Verification items for this drawing (mm, ordinates from the low corner). Round coordinates to 2 decimals unless told otherwise and drop trailing zeros. Order: outer loops, then holes, each group sorted by start corner. A loop starts at its lowest first (then second) coordinate and runs counter-clockwise, first axis right, second up. Notation, with made-up numbers: (-16.5, 12) -> (28.5, 12) arc R22 cw to (28.5, 22) -> close; hole circle Ø4 at (-6, 75). An arc over 180 degrees is marked (long way). Return JSON: item names as keys, results as strings. Group by question number.
Item 1: Sectioned sample at A-A on x = 4. Record the cut outline in (y, z), plus the area to 3 significant figures.
Item 2: Sectioned sample at B-B on z = 0.65. Record the cut outline in (x, y).
Item 3: Sectioned sample at C-C on y = 69.5. Record the cut outline in (x, z).
Item 4: Scan lines: probe 1 along Y at (x, z) = (4.25, 0.4); probe 2 along X at (y, z) = (4, 0.7); probe 3 along X at (y, z) = (73, 0.35). Record each from-to range of solid material in increasing order. Write a range as from..to.
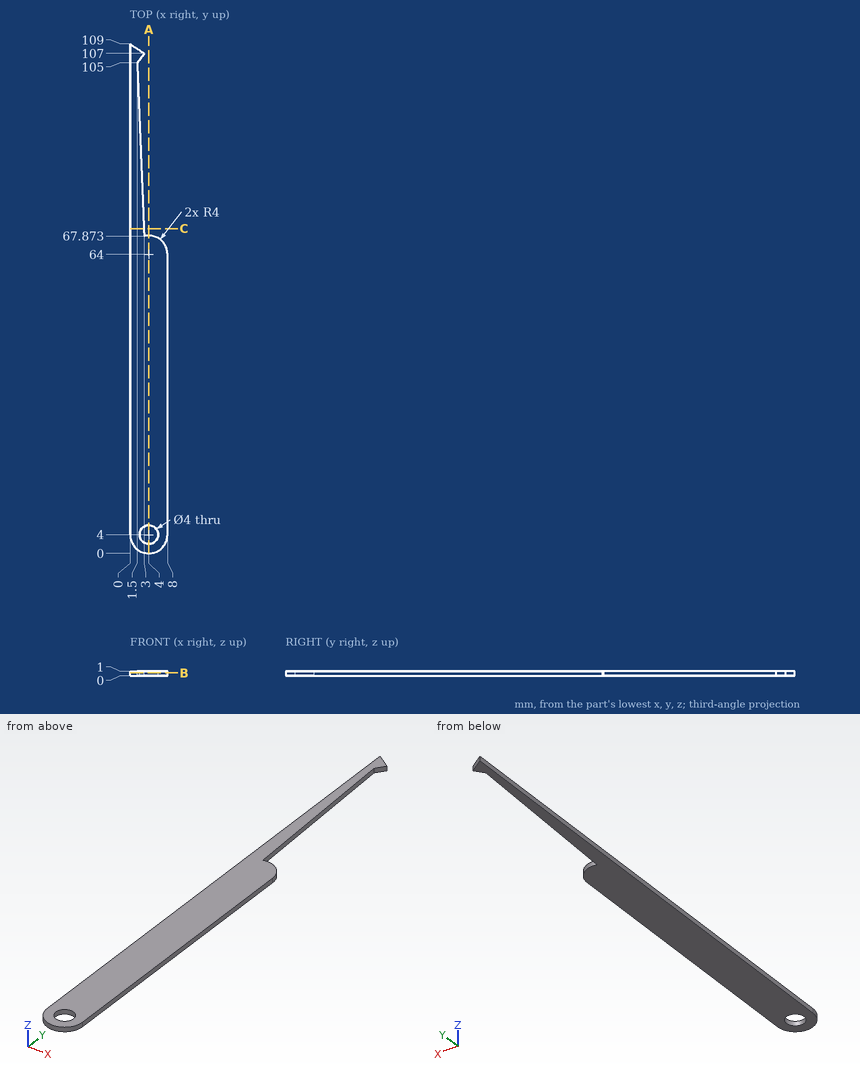
Recorded:
{
 "1": {"outline": "(0, 0) -> (2, 0) -> (2, 1) -> (0, 1) -> close; (6, 0) -> (68, 0) -> (68, 1) -> (6, 1) -> close", "area": "64.0 mm²"},
 "2": {"outline": "(0, 4) arc R4 ccw to (8, 4) -> (8, 64) arc R4 ccw to (3, 67.87) -> (1.5, 105) -> (3, 107) -> (0, 109) -> close; hole circle Ø4 at (4, 4)"},
 "3": {"outline": "(0, 0) -> (2.93, 0) -> (2.93, 1) -> (0, 1) -> close"},
 "4": {"probe 1": "0.01..2.02, 5.98..67.99", "probe 2": "0..2, 6..8", "probe 3": "0..2.79"}
}
